Here's how the part is built. I have some questions about the finished solid (model axes, mm). Face numbers are marked on the shaded views. A direction names the side the tool comes from. Round coordinates to 2 decimals unless told otherwise and drop trailing zeros. Order: outer loops, then holes, each group sorted by start corner. A loop starts at its lowest first (then second) coordinate and runs counter-clockwise, first axis right, second up. Notation, with made-up numbers: (16, 70.25) -> (21, 70.25) arc R12 cw to (21, 82.25) -> close; hole circle Ø5 at (70.5, -4.5). An arc over 180 degrees is marked (long way). Use a Markdown table: item, result. Add a question column.
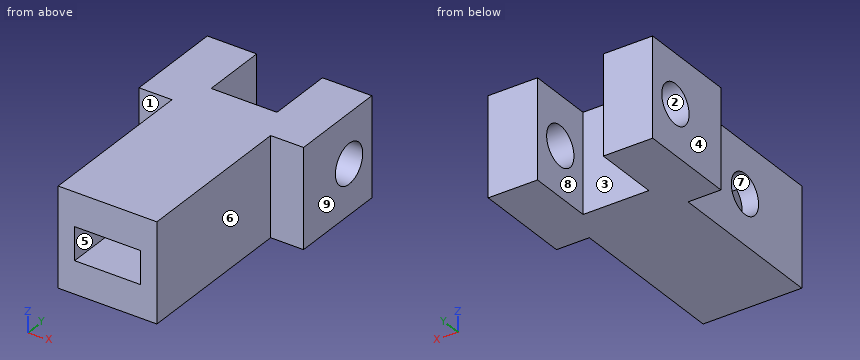
from build123d import *

# Parameters (mm, degrees)
BOSS_EXTRUDE1_DEPTH = 15
SKETCH2_R           = 3
CUT_EXTRUDE1_DEPTH  = 35
SKETCH3_W           = 15
SKETCH3_H           = 15
SKETCH3_W_2         = 10
SKETCH3_H_2         = 5
BOSS_EXTRUDE2_DEPTH = 25
SKETCH5_R           = 3
CUT_EXTRUDE3_DEPTH  = 7


with BuildPart() as part:
    # Sketch1 → Boss-Extrude1 (new body)
    with BuildSketch(Plane.XY):
        Polygon((3.687581296, 3.934802907), (3.687581296, -6.065197093), (-6.312418704, -6.065197093), (-6.312418704, 3.934802907), (-13.812418704, 3.934802907), (-13.812418704, -11.065197093), (11.187581296, -11.065197093), (11.187581296, 3.934802907), align=None)
    extrude(amount=BOSS_EXTRUDE1_DEPTH)

    # Sketch2 → Cut-Extrude1 (cut)
    with BuildSketch(Plane(origin=(11.187581296, 0, 0), x_dir=(0, 0, -1), z_dir=(1, 0, 0))):
        with Locations(Location((-7.534884308, -1.065197093, 0), (0, 0, 90))):
            Circle(SKETCH2_R)
    extrude(amount=-CUT_EXTRUDE1_DEPTH, mode=Mode.SUBTRACT)

    # Sketch3 → Boss-Extrude2 (add)
    with BuildSketch(Plane.XZ.offset(11.065197093)):
        with Locations((-1.312418704, 7.5)):
            Rectangle(SKETCH3_W, SKETCH3_H)
        with Locations((-1.312418704, 7.415567581)):
            Rectangle(SKETCH3_W_2, SKETCH3_H_2, mode=Mode.SUBTRACT)
    extrude(amount=BOSS_EXTRUDE2_DEPTH)

    # Sketch5 → Cut-Extrude3 (cut)
    with BuildSketch(Plane.ZY.offset(8.812418704)):
        with Locations((7.5, -23.565197093)):
            Circle(SKETCH5_R)
    extrude(amount=-CUT_EXTRUDE3_DEPTH, mode=Mode.SUBTRACT)


solid = part.part
(1) If we mould it in two halves opening along Y, with no side actions, what happens to the marked faces 1, 2, 3 and 4? For each: pulls with the +Y half, pulls with the -Y half, needs draft (parallel to the pull), parting line crosses it, or undercut.
(2) I want a section at D-D on z = 3. List the corners of the cut face in (x, y) for me.
(3) I want a section at B-B on z = 9. List the corners of the cut face in (x, y) for me.
(4) Please list where these lines run through material, in increasing order: probe 1 along Y at (x, z) = (-6.5, 7.5) (3 decimals); probe 2 along Z at (x, y) = (1, -22); probe 3 along X at (y, z) = (-31, 7). Write a range as from..to.
(5) I want a section at A-A on y = -14.5. List the corners of the cut face in (x, z) for me.
(6) I'm going to push flat-ended pins straight in: P1, Ø2.5, axis at x = 0, z = 7.5, coming from the -Y side; P2, Ø1.5, axis at y = -16, z = 13.5, coming from the +X side; P3, Ø6, axis at y = -27.5, z = 7, coming from the -X side. Where does each tip first touch, or does it pass through?
(7) I want a section at C-C on x = 0. List the corners of the cut face in (y, z) for me.
(8) On a 3-axis mill with a long thin cutter (end or side, diameter ignored), from which of +Z, -Z, +X, -X, +Y, -Y can I reach the whole of each face in a straight line? I mean the marked faces 5, 6, 7, 8 and 9. Say none if no direction works.
Output:
| question | item | result |
|---|---|---|
| 1 | face 1 | pulls with the -Y half |
| 1 | face 2 | undercut |
| 1 | face 3 | pulls with the +Y half |
| 1 | face 4 | needs draft |
| 2 | outline | (-13.81, -11.07) -> (-8.81, -11.07) -> (-8.81, -36.07) -> (6.19, -36.07) -> (6.19, -11.07) -> (11.19, -11.07) -> (11.19, 3.93) -> (3.69, 3.93) -> (3.69, -6.07) -> (-6.31, -6.07) -> (-6.31, 3.93) -> (-13.81, 3.93) -> close |
| 3 | outline | (-13.81, -11.07) -> (-8.81, -11.07) -> (-8.81, -20.97) -> (-6.31, -20.97) -> (-6.31, -11.07) -> (3.69, -11.07) -> (3.69, -36.07) -> (6.19, -36.07) -> (6.19, -11.07) -> (11.19, -11.07) -> (11.19, -3.68) -> (3.69, -3.68) -> (3.69, -6.07) -> (-6.31, -6.07) -> (-6.31, -3.68) -> (-13.81, -3.68) -> close; (-13.81, 1.55) -> (-6.31, 1.55) -> (-6.31, 3.93) -> (-13.81, 3.93) -> close; (-8.81, -36.07) -> (-6.31, -36.07) -> (-6.31, -26.16) -> (-8.81, -26.16) -> close; (3.69, 1.55) -> (11.19, 1.55) -> (11.19, 3.93) -> (3.69, 3.93) -> close |
| 4 | probe 1 | -36.065..-26.565, -20.565..-4.065, 1.935..3.935 |
| 4 | probe 2 | 0..4.92, 9.92..15 |
| 4 | probe 3 | -8.81..-6.31, 3.69..6.19 |
| 5 | outline | (-8.81, 0) -> (6.19, 0) -> (6.19, 15) -> (-8.81, 15) -> close; hole (-6.31, 4.92) -> (3.69, 4.92) -> (3.69, 9.92) -> (-6.31, 9.92) -> close |
| 6 | P1 | y = -11.07 |
| 6 | P2 | x = 6.19 |
| 6 | P3 | x = -8.81 |
| 7 | outline | (-36.07, 0) -> (-6.07, 0) -> (-6.07, 15) -> (-36.07, 15) -> (-36.07, 9.92) -> (-11.07, 9.92) -> (-11.07, 4.92) -> (-36.07, 4.92) -> close |
| 8 | face 5 | -Y |
| 8 | face 6 | +Z, -Z, +X, -Y |
| 8 | face 7 | -X |
| 8 | face 8 | +Z, -Z, +Y |
| 8 | face 9 | +Z, -Z, +X, +Y, -Y |
